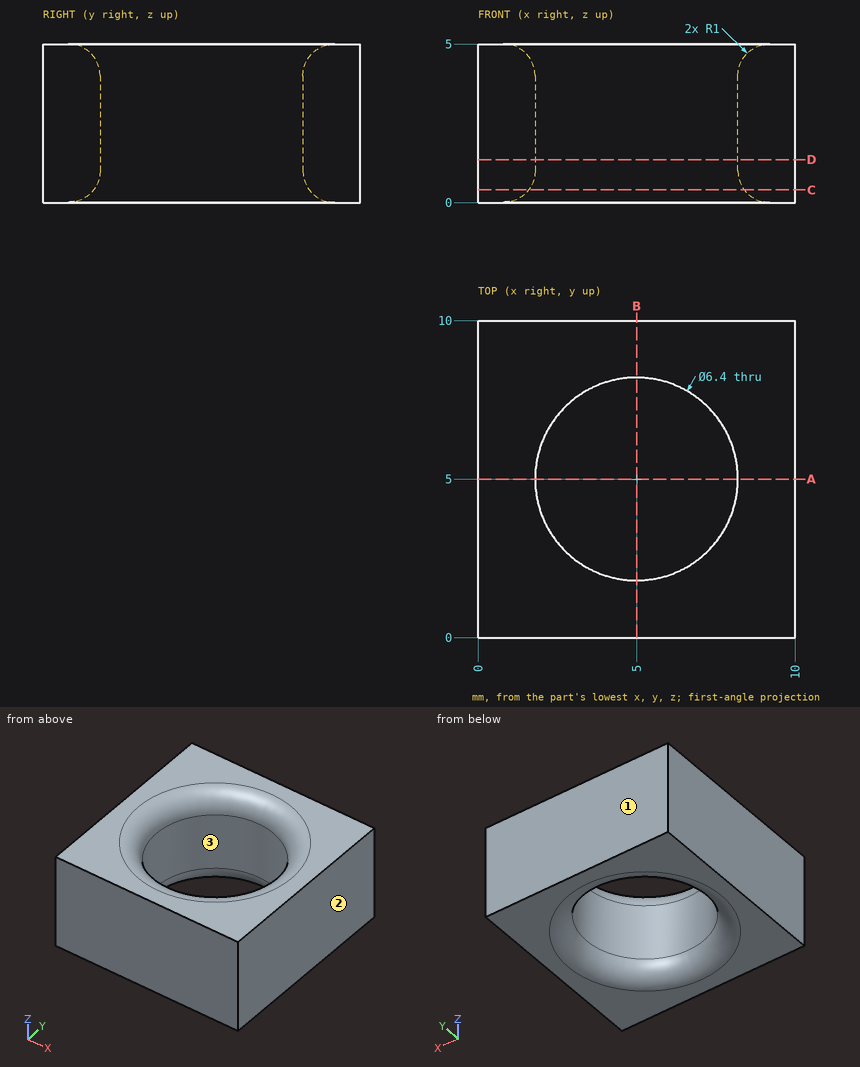
Check sheet for the drawn part. Datum: minimum x, y, z corner. Units: mm. Round coordinates to 2 decimals unless told otherwise and drop trailing zeros. Order: outer loops, then holes, each group sorted by start corner. A loop starts at its lowest first (then second) coordinate and runs counter-clockwise, first axis right, second up. Notation, with made-up numbers: (-11.5, 73.5) -> (21.5, 73.5) arc R23 cw to (21.5, 104.5) -> close; hole circle Ø1 at (-7.75, 62.5). An arc over 180 degrees is marked (long way). Return JSON: item names as keys, results as strings. Group by question number.
Q1. Section check C-C, the plane z = 0.4. Record the boundary of the cut face in (x, y).
Q2. Release check for a two-part mould opening along Y. For the marked faces 1, 2 and 3 record: released by +Y, released by -Y, zero draft, split by the parting line, or undercut.
Q3. Section check A-A, the plane y = 5. Record the boundary of the cut face in (x, z).
Q4. Gauge pin test, flat ends, axial feed: pin 1 (2 mm diameter, centred on x = 3, y = 8.5, fed in from +Z); pin 2 (5 mm diameter, centred on x = 5, y = 5, fed in from +Z). Record the tip position at first contact, or that the pin passes through.
Q5. Section check D-D, the plane z = 1.35. Record the boundary of the cut face in (x, y), plus the area to 3 significant figures.
Q6. Material ranges on probe 1 along Y at (x, z) = (5, 3.1); probe 2 along Y at (x, z) = (7.25, 2.6); probe 3 along X at (y, z) = (2.25, 2.2), recorded low to high. Write a range as from..to.
Numbers:
{
 "1": {"outline": "(0, 0) -> (10, 0) -> (10, 10) -> (0, 10) -> close; hole circle Ø6.8 at (5, 5)"},
 "2": {"face 1": "released by +Y", "face 2": "zero draft", "face 3": "undercut"},
 "3": {"outline": "(0, 0) -> (0.8, 0) arc R1 ccw to (1.8, 1) -> (1.8, 4) arc R1 ccw to (0.8, 5) -> (0, 5) -> close; (8.2, 1) arc R1 ccw to (9.2, 0) -> (10, 0) -> (10, 5) -> (9.2, 5) arc R1 ccw to (8.2, 4) -> close"},
 "4": {"pin 1": "z = 5", "pin 2": "through"},
 "5": {"outline": "(0, 0) -> (10, 0) -> (10, 10) -> (0, 10) -> close; hole circle Ø6.4 at (5, 5)", "area": "67.8 mm^2"},
 "6": {"probe 1": "0..1.8, 8.2..10", "probe 2": "0..2.72, 7.28..10", "probe 3": "0..3.36, 6.64..10"}
}
